Autodesk Inventor part; units mm, degrees
ref_plane "ANBAU_XY" through (0, 0, 0) normal (0, 0, 1) x (1, 0, 0)
ref_plane "ANBAU_YZ" through (0, 0, 0) normal (1, 0, 0) x (0, 1, 0)
ref_plane "ANBAU_ZX" through (0, 0, 0) normal (0, 1, 0) x (0, 0, 1)
sketch "Sketch_1" plane through (0, 0, 0) normal (1, 0, 0) x (0, 1, 0)
  line L0 (0, -3.8) -> (0, 1.634)
  line L1 (0, 1.634) -> (1.5, 2.5)
  line L2 (1.5, 2.5) -> (3.8, 2.5)
  arc A0 (4, 2.3) -> (3.8, 2.5) centre (3.8, 2.3) ccw
  line L3 (4, 2.3) -> (4, 0.8333)
  line L4 (4, 0.8333) -> (3.6, 0.8333)
  line L5 (3.6, 0.8333) -> (3.6, 0.6833)
  line L6 (3.6, 0.6833) -> (4, 0.6833)
  line L7 (4, 0.6833) -> (4, 0)
  line L8 (4, 0) -> (2.0095, 0)
  line L9 (2.0095, 0) -> (2.5, -0.4905)
  line L10 (2.5, -0.4905) -> (2.5, -3.3095)
  line L11 (2.5, -3.3095) -> (2.0095, -3.8)
  line L12 (2.0095, -3.8) -> (0, -3.8)
  line L13 (0, -3.8) -> (0, 1.634)
revolve "Revolution1" add sketch "Sketch_1" angle 360 about axis through (0, 0, -3.8) along (0, 0, -1)
thread "Thread1"
sketch "Skizze_4" plane through (0, 0, 2.5) normal (0, 0, 1) x (1, 0, 0)
  line L0 (-1.25, -0.7217) -> (0, -1.4434)
  line L1 (0, -1.4434) -> (1.25, -0.7217)
  line L2 (1.25, -0.7217) -> (1.25, 0.7217)
  line L3 (1.25, 0.7217) -> (0, 1.4434)
  line L4 (0, 1.4434) -> (-1.25, 0.7217)
  line L5 (-1.25, 0.7217) -> (-1.25, -0.7217)
extrude "Extrusion1" cut sketch "Skizze_4" against normal blind 2.5
ref_plane "ANBAU_XY" through (0, 0, 0) normal (0, 0, 1) x (1, 0, 0)
ref_plane "ANBAU_YZ" through (0, 0, 0) normal (1, 0, 0) x (0, 1, 0)
ref_plane "ANBAU_ZX" through (0, 0, 0) normal (0, 1, 0) x (0, 0, 1)
ref_plane "ANBAU_STD_XY" through (0, 0, 0) normal (0, 0, 1) x (1, 0, 0)
ref_plane "ANBAU_STD_YZ" through (0, 0, 0) normal (1, 0, 0) x (0, 1, 0)
ref_plane "ANBAU_STD_ZX" through (0, 0, 0) normal (0, 1, 0) x (0, 0, 1)
ref_plane "CPV_XY" through (0, 0, 0) normal (0, 0, 1) x (1, 0, 0)
ref_plane "CPV_YZ" through (0, 0, 0) normal (1, 0, 0) x (0, 1, 0)
ref_plane "CPV_ZX" through (0, 0, 0) normal (0, 1, 0) x (0, 0, 1)
properties part number "174308 B-M5-B"
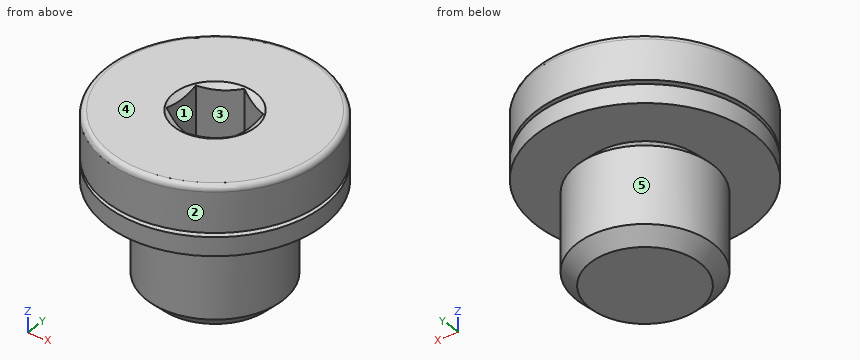
Can you work these out from the model? Positions are in its coordinate system, mm. Face numbers are marked on the shaded views. A direction names the side the tool comes from. Round coordinates to 2 decimals unless told otherwise and drop trailing zeros. Loops run counter-clockwise (first coordinate to the right, second up) from the corner with the lowest first, then second, coordinate; pieces in that order, holes last. Notation, with made-up numbers: M 62,60.25 L 79,60.25 A25 cw 79,86.25 Z; hole C -33,18.25 d9. An arc over 180 degrees is marked long. Answer in a Markdown table with one row per item.
1. If we section it at C-C, the plane z = -3.5: Please give me the cut outline in (x, y), plus the area to 3 significant figures.
Established:
| item | result |
|---|---|
| outline | C 0,0 d4.62 |
| area | 16.8 mm² |
2. Please list where these lines run through material, in increasing order: line 1 (Z direction, x = -1.75, y = -3.5); line 2 (Z direction, x = -1.75, y = 3); line 3 (Y direction, x = -2, z = -2.25). Write a range as from..to.
Established:
| item | result |
|---|---|
| line 1 | 0..0.68, 0.83..2.46 |
| line 2 | 0..2.5 |
| line 3 | -1.5..1.5 |
3. If we section it at A-A, the plane y = 0: Please give me the cut outline in (x, z), plus the area to 3 significant figures.
Established:
| item | result |
|---|---|
| outline | M -4,0 L -2.01,0 L -2.5,-0.49 L -2.5,-3.31 L -2.01,-3.8 L 2.01,-3.8 L 2.5,-3.31 L 2.5,-0.49 L 2.01,0 L 4,0 L 4,0.68 L 3.6,0.68 L 3.6,0.83 L 4,0.83 L 4,2.3 A0.2 ccw 3.8,2.5 L 1.5,2.5 L 1.25,2.36 L 1.25,0 L -1.25,0 L -1.25,2.36 L -1.5,2.5 L -3.8,2.5 A0.2 ccw -4,2.3 L -4,0.83 L -3.6,0.83 L -3.6,0.68 L -4,0.68 Z |
| area | 32.1 mm² |
4. Thinking about a two-plate mould opening in Y: for the marked faces 3, 4 and 5, which applies, pulls with the +Y half, pulls with the -Y half, needs draft (parallel to the pull), parting line crosses it, or undercut?
Established:
| item | result |
|---|---|
| face 3 | undercut |
| face 4 | needs draft |
| face 5 | parting line crosses it |
5. If we section it at B-B, the plane z = -0.75: Please give me the cut outline in (x, y), plus the area to 3 significant figures.
Established:
| item | result |
|---|---|
| outline | C 0,0 d5 |
| area | 19.6 mm² |
6. I'm going to push flat-ended pins straight in: pin 1 Ø3 at (x, z) = (-3, -0.5) entering from +Y; pin 2 Ø1 at (x, y) = (2, 3) entering from -Z. Where does each tip first touch, or does it pass through?
Established:
| item | result |
|---|---|
| pin 1 | y = 3.67 |
| pin 2 | z = 0 |
7. On a 3-axis mill with a long thin cutter (end or side, diameter ignored), from which of +Z, -Z, +X, -X, +Y, -Y can I reach the whole of each face in a straight line? I mean the marked faces 1 and 2. Say none if no direction works.
Established:
| item | result |
|---|---|
| face 1 | +Z |
| face 2 | +Z, -Z |
